Design review of the part shown in the three views and the two pictorial views. Dimensions are in mm from the part's minimum x, y and z. A direction names the side the tool comes from. Coordinates: 2 decimals unless noted, no trailing zeros. Loops run counter-clockwise (first coordinate to the right, second up) from the corner with the lowest first, then second, coordinate; pieces in that order, holes last. Notation, with made-up numbers: (-19.75, 33.25) -> (23.25, 33.25) arc R14 ccw to (23.25, 45.25) -> close; hole circle Ø11 at (-23.75, 42). An arc over 180 degrees is marked (long way). One line per item, written item: value.
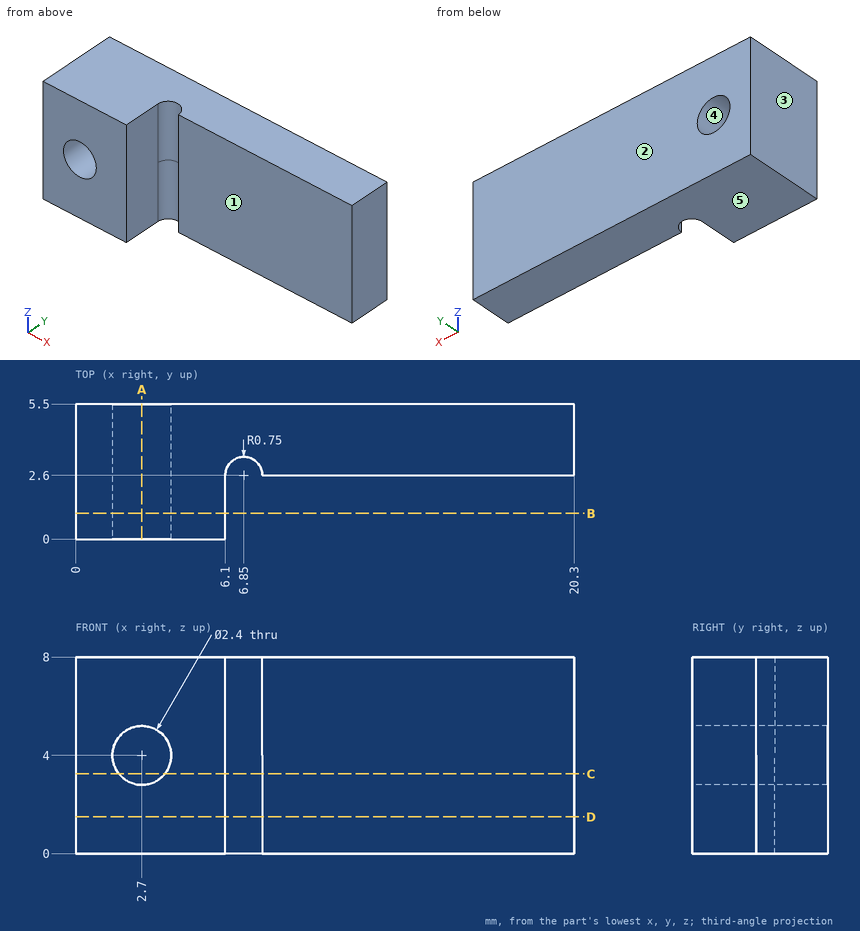
1. Take a section at D-D, the plane z = 1.5. Give the boundary of the cut face in (x, y).
Return value:
outline: (0, 0) -> (6.1, 0) -> (6.1, 2.6) arc R0.75 cw to (7.6, 2.6) -> (20.3, 2.6) -> (20.3, 5.5) -> (0, 5.5) -> close
2. Take a section at B-B, the plane y = 1.05. Give the boundary of the cut face in (x, z), and give its area (3 significant figures).
Return value:
outline: (0, 0) -> (6.1, 0) -> (6.1, 8) -> (0, 8) -> close; hole circle Ø2.4 at (2.7, 4)
area: 44.3 mm2
3. Take a section at A-A, the plane x = 2.7. Give the boundary of the cut face in (y, z), and give its area (3 significant figures).
Return value:
outline: (0, 0) -> (5.5, 0) -> (5.5, 2.8) -> (0, 2.8) -> close; (0, 5.2) -> (5.5, 5.2) -> (5.5, 8) -> (0, 8) -> close
area: 30.8 mm2
4. Take a section at C-C, the plane z = 3.25. Give the boundary of the cut face in (x, y), and give its area (3 significant figures).
Return value:
outline: (0, 0) -> (1.76, 0) -> (1.76, 5.5) -> (0, 5.5) -> close; (3.64, 0) -> (6.1, 0) -> (6.1, 2.6) arc R0.75 cw to (7.6, 2.6) -> (20.3, 2.6) -> (20.3, 5.5) -> (3.64, 5.5) -> close
area: 63.5 mm2
5. Insertion check: pin 1 Ø3 at (y, z) = (1, 4.5) entering from +X; pin 2 Ø4 at (x, z) = (16, 3.5) entering from -Y. Each pin has a flat end and moves straight along its axis. Give the tip position at first contact, or say it passes through.
Return value:
pin 1: stops at x = 6.1
pin 2: stops at y = 2.6
6. For the marked faces 1 and 2, list the 3-axis set-ups (+Z, -Z, +X, -X, +Y, -Y) from which the entire face can be reached by the end or side of a thin tool; tool diameter is ignored.
Return value:
face 1: +Z, -Z, +X, -Y
face 2: +Z, -Z, +X, -X, +Y
7. To check wall thickness, follow probe 1 along Z at (x, y) = (2.7, 1.2); probe 2 along X at (y, z) = (4.05, 4); probe 3 along X at (y, z) = (1.7, 4). State the ranges of each line that lie inside material, in increasing order. Write a range as from..to.
Return value:
probe 1: z = 0..2.8, 5.2..8
probe 2: x = 0..1.5, 3.9..20.3
probe 3: x = 0..1.5, 3.9..6.1
8. The part is to be moulded in two halves that separate along X. For the marked faces 3, 4 and 5, say which applies: pulls with the +X half, pulls with the -X half, needs draft (parallel to the pull), parting line crosses it, or undercut.
Return value:
face 3: pulls with the -X half
face 4: undercut
face 5: needs draft
